from build123d import *

# Parameters (mm, degrees)
PAD_DEPTH    = 20
SKETCH001_R  = 4
POCKET_DEPTH = 20


with BuildPart() as part:
    # Sketch → Pad (new body)
    with BuildSketch(Plane.YZ):
        Polygon((-30, -5), (30, -5), (30, 5), (10, 5), (10, 45), (-10, 45), (-10, 5), (-30, 5), align=None)
    extrude(amount=PAD_DEPTH)

    # Sketch001 → Pocket (cut)
    with BuildSketch(Plane.YZ.offset(20)):
        with Locations((0, 35)):
            Circle(SKETCH001_R)
        with Locations((0, 19)):
            Circle(SKETCH001_R)
    extrude(amount=-POCKET_DEPTH, mode=Mode.SUBTRACT)


solid = part.part
Design review of the part built by this model. Coordinates are the model's own, in mm. A direction names the side the tool comes from. Round coordinates to 2 decimals unless told otherwise and drop trailing zeros. Order: outer loops, then holes, each group sorted by start corner. A loop starts at its lowest first (then second) coordinate and runs counter-clockwise, first axis right, second up.
1) Consider section D-D (z = 27). State the section outline as (x, y) points.
The answers:
outline: (0, -10) - (20, -10) - (20, 10) - (0, 10) - close
2) Machinability: for faces 5 (the flat face through (10, 20, 5)), 6 (the flat face through (0, -0.4, 14.8)), 7 (the flat face through (10, -20, 5)), which of the approach directions +Z, -Z, +X, -X, +Y, -Y give a long, thin tool a straight path to every point of the face, cutting with its end or side? Answer none if there is none.
The answers:
face 5: +Z, +X, -X, +Y
face 6: +Z, -Z, -X, +Y, -Y
face 7: +Z, +X, -X, -Y
3) For L1, parallel to Z at x = 11.5, y = 0; L2, parallel to Z at x = 18.25, y = -1.5; L3, parallel to Y at x = 7.5, z = 42, list the stretches that pass through material, from the lowest coordinate up.
The answers:
L1: z = -5 to 15, 23 to 31, 39 to 45
L2: z = -5 to 15.29, 22.71 to 31.29, 38.71 to 45
L3: y = -10 to 10
4) Consider section C-C (y = 0). State the section outline as (x, z) points.
The answers:
outline: (0, -5) - (20, -5) - (20, 15) - (0, 15) - close; (0, 23) - (20, 23) - (20, 31) - (0, 31) - close; (0, 39) - (20, 39) - (20, 45) - (0, 45) - close
5) Consider section B-B (z = 19). State the section outline as (x, y) points.
The answers:
outline: (0, -10) - (20, -10) - (20, -4) - (0, -4) - close; (0, 4) - (20, 4) - (20, 10) - (0, 10) - close
6) Draft analysis for pull direction Y (two halves, no side actions). For faces 1 (the flat face through (10, 10, 25)), 2 (the cylindrical face through (10.14, -0.521, 22.966)), 3 (the cylindrical face through (10.14, -0.521, 38.966)), 4 (the flat face through (10, -10, 25)), state which applies: released by +Y, released by -Y, zero draft, split by the parting line, or undercut.
The answers:
face 1: released by +Y
face 2: undercut
face 3: undercut
face 4: released by -Y
7) Clearance check with flat-ended pins moving along their axes: pin 1 Ø4 at (x, y) = (9, 22.5) entering from +Z; pin 2 Ø12 at (x, z) = (14.5, 34) entering from -Y; pin 3 Ø10 at (x, z) = (9, 33.5) entering from +Y. State where each tip first meets the part, or that it passes through.
The answers:
pin 1: stops at z = 5
pin 2: stops at y = -10
pin 3: stops at y = 10
8) Consider section A-A (x = 1.5). State the section outline as (y, z) points.
The answers:
outline: (-30, -5) - (30, -5) - (30, 5) - (10, 5) - (10, 45) - (-10, 45) - (-10, 5) - (-30, 5) - close; hole circle Ø8 at (0, 19); hole circle Ø8 at (0, 35)
